Input: part model. Units: mm. Frame: model coordinates. A direction names the side the tool comes from. Give positions to 0.01 mm unless a question says otherwise; leave off trailing zeros. Order: outer loops, then holes, each group sorted by start corner. A loop starts at its lowest first (then second) coordinate and runs counter-clockwise, first axis right, second up. Notation, with made-up numbers: (81, 38.25) - (132, 38.25) arc R15 ccw to (132, 42.25) - close; hole circle Ø5 at (69, -16.5). An arc over 180 degrees is marked (long way). Answer in a Markdown table with one row per item. Add a question column.
1. Section query B-B on y = 6. Return loops of the section in (x, z).
2. Mould query, pull axis X, two halves, no side actions, for faces 5 (the face through (-37.5, 14, -6)), 6 (the face through (-25, 6, 25)), 7 (the face through (0, 6, 9.511)). Classes: released by +X, released by -X, zero draft, split by the parting line, or undercut.
3. Ray query, line 1 (X direction, y = 11, z = 12); line 2 (Y direction, x = -17.5, z = -3); line 3 (Z direction, x = -10.5, y = 7). Return the intervals inside material, ascending. Write a range as [from, to].
4. Access query for faces 1 (the face through (9, 12, 5)), 2 (the face through (-12.5, 6, 17)), 3 (the face through (-16, 22, -5)), 4 (the face through (-28, 37, -15)). Directions: +Z, -Z, +X, -X, +Y, -Y. A direction counts if a zero-diameter tool reaches every point of the face in a straight line with its end or side. Return the directions, or none.
5. Section query C-C on x = 0. Return loops of the section in (y, z), and give its area (3 significant figures).
6. Section query D-D on z = -16.5. Return loops of the section in (x, y), and give its area (3 significant figures).
7. Section query A-A on z = 11. Return loops of the section in (x, y), and give its area (3 significant figures).
8. Contact query for flat-ended pins moving along their axis: pin 1 (10 mm diameter, centred on x = 23.5, z = 5.5, fed in from +Y); pin 2 (5 mm diameter, centred on x = -24.5, y = 27, fed in from +Z); pin 3 (9.5 mm diameter, centred on x = 4, y = 8, fed in from +Z). Output: stop coordinate, or through.
```python
from build123d import *

# Parameters (mm, degrees)
BOSS_EXTRUDE1_DEPTH = 12
BOSS_EXTRUDE4_DEPTH = 20


with BuildPart() as part:
    # Sketch2 → Boss-Extrude1 (new body)
    with BuildSketch(Plane(origin=(0, 0, 0), x_dir=(1, 0, 0), z_dir=(0, 1, 0))):
        Polygon((-37.5, 25), (37.5, 25), (37.5, -25), (12.5, -25), (12.5, -9.510869565), (-12.5, -9.510869565), (-12.5, -25), (-37.5, -25), align=None)
    extrude(amount=BOSS_EXTRUDE1_DEPTH)

    # Sketch4 → Boss-Extrude4 (add)
    with BuildSketch(Plane(origin=(0, 0, -25), x_dir=(-1, 0, 0), z_dir=(0, 0, -1))):
        Polygon((37.5, 12), (37.5, 37), (17.5, 37), (-17.5, 12), align=None)
    extrude(amount=-BOSS_EXTRUDE4_DEPTH)


solid = part.part
```
Answer:
| question | item | result |
|---|---|---|
| 1 | outline | (-37.5, -25) - (37.5, -25) - (37.5, 25) - (12.5, 25) - (12.5, 9.51) - (-12.5, 9.51) - (-12.5, 25) - (-37.5, 25) - close |
| 2 | face 5 | released by -X |
| 2 | face 6 | zero draft |
| 2 | face 7 | undercut |
| 3 | line 1 | x = [-37.5, -12.5], [12.5, 37.5] |
| 3 | line 2 | y = [0, 12] |
| 3 | line 3 | z = [-25, 9.51] |
| 4 | face 1 | +Z, +X, +Y |
| 4 | face 2 | +Z, +Y, -Y |
| 4 | face 3 | +Z, +X, -X, +Y |
| 4 | face 4 | +Z, -Z, +X, -X, +Y |
| 5 | outline | (0, -25) - (24.5, -25) - (24.5, -5) - (12, -5) - (12, 9.51) - (0, 9.51) - close |
| 5 | area | 664 mm² |
| 6 | outline | (-37.5, 0) - (37.5, 0) - (37.5, 12) - (17.5, 12) - (-17.5, 37) - (-37.5, 37) - close |
| 6 | area | 1,840 mm² |
| 7 | outline | (-37.5, 0) - (-12.5, 0) - (-12.5, 12) - (-37.5, 12) - close; (12.5, 0) - (37.5, 0) - (37.5, 12) - (12.5, 12) - close |
| 7 | area | 600 mm² |
| 8 | pin 1 | stops at y = 12 |
| 8 | pin 2 | stops at z = -5 |
| 8 | pin 3 | stops at z = 9.51 |
